```python
from build123d import *

# Parameters (mm, degrees)
SKETCH_1_W      = 28
SKETCH_1_H      = 8.6
SKETCH_1_W_2    = 26
SKETCH_1_H_2    = 6.6
EXTRUDE_1_DEPTH = 1
SKETCH_2_W      = 30
SKETCH_2_H      = 10
SKETCH_2_W_2    = 26
SKETCH_2_H_2    = 6.54302186
EXTRUDE_2_DEPTH = 0.5


with BuildPart() as part:
    # Эскиз1 → Бобышка-Вытянуть1 (new body)
    with BuildSketch(Plane.XY):
        with Locations((-21.588376798, -20.389004385)):
            Rectangle(SKETCH_1_W, SKETCH_1_H)
        with Locations((-21.588376798, -20.389004385)):
            Rectangle(SKETCH_1_W_2, SKETCH_1_H_2, mode=Mode.SUBTRACT)
    extrude(amount=-EXTRUDE_1_DEPTH)

    # Эскиз2 → Бобышка-Вытянуть2 (add)
    with BuildSketch(Plane.XY):
        with Locations((-21.588376798, -20.289004385)):
            Rectangle(SKETCH_2_W, SKETCH_2_H)
        with Locations((-21.588376798, -20.360515315)):
            Rectangle(SKETCH_2_W_2, SKETCH_2_H_2, mode=Mode.SUBTRACT)
    extrude(amount=EXTRUDE_2_DEPTH)


solid = part.part
```
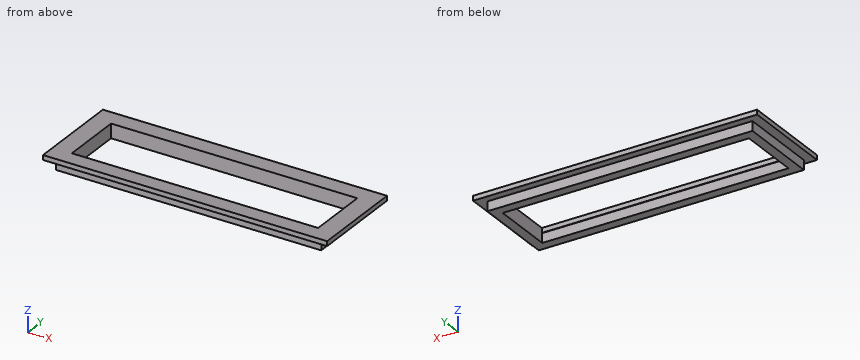
Input: part model. Units: mm. Frame: model coordinates. Coordinates: 2 decimals unless noted, no trailing zeros. Write each loop counter-clockwise with the first axis right and the second up, starting at its lowest first coordinate (ties: lowest second). Pieces come first, ordered by that corner, then holes. Notation, with made-up numbers: (47.25, 58.25) -> (57.25, 58.25) arc R10 ccw to (57.25, 74.25) -> close; hole circle Ø3 at (9.25, -8). An arc over 180 degrees is marked (long way). Answer as a JSON object with one key per item and string values.
1. First-contact query: P1, Ø0.8, axis at x = -27.5, z = -0.5, coming from the -Y side; P2, Ø0.8, axis at x = -20, z = -0.5, coming from the +Y side; P3, Ø0.8, axis at y = -20, z = -0.5, coming from the +X side. Flat tips, straight axial feed; report the tip coordinate or a pass-through.
Result set:
{"P1": "stops at y = -24.69", "P2": "stops at y = -16.09", "P3": "stops at x = -7.59"}
2. Section A-A on x = -11.75. Return the cut outline in (y, z), then the cut area to 3 significant figures.
Result set:
{"outline": "(-25.29, 0) -> (-24.69, 0) -> (-24.69, -1) -> (-23.69, -1) -> (-23.69, 0) -> (-23.63, 0) -> (-23.63, 0.5) -> (-25.29, 0.5) -> close; (-17.09, -1) -> (-16.09, -1) -> (-16.09, 0) -> (-15.29, 0) -> (-15.29, 0.5) -> (-17.09, 0.5) -> close", "area": "3.73 mm2"}
3. Section D-D on y = -15.75. Return the cut outline in (x, z), then the cut area to 3 significant figures.
Result set:
{"outline": "(-36.59, 0) -> (-6.59, 0) -> (-6.59, 0.5) -> (-36.59, 0.5) -> close", "area": "15.0 mm2"}
4. Section C-C on z = -0.25. Return the cut outline in (x, y), then the cut area to 3 significant figures.
Result set:
{"outline": "(-35.59, -24.69) -> (-7.59, -24.69) -> (-7.59, -16.09) -> (-35.59, -16.09) -> close; hole (-34.59, -23.69) -> (-8.59, -23.69) -> (-8.59, -17.09) -> (-34.59, -17.09) -> close", "area": "69.2 mm2"}
5. Section B-B on y = -22. Return the cut outline in (x, z), then the cut area to 3 significant figures.
Result set:
{"outline": "(-36.59, 0) -> (-35.59, 0) -> (-35.59, -1) -> (-34.59, -1) -> (-34.59, 0.5) -> (-36.59, 0.5) -> close; (-8.59, -1) -> (-7.59, -1) -> (-7.59, 0) -> (-6.59, 0) -> (-6.59, 0.5) -> (-8.59, 0.5) -> close", "area": "4.00 mm2"}
6. Material intervals for line 1 (Y direction, x = -16.5, z = 0.2); line 2 (Y direction, x = -31.5, z = -0.15); line 3 (X direction, y = -18.25, z = 0.1), sorted ascending. Write a range as from..to.
Result set:
{"line 1": "y = -25.29..-23.63, -17.09..-15.29", "line 2": "y = -24.69..-23.69, -17.09..-16.09", "line 3": "x = -36.59..-34.59, -8.59..-6.59"}
